Geometry check sheet. Reference: drawing and pictorial views, mm from the part's lowest x, y, z. Round coordinates to 2 decimals unless told otherwise and drop trailing zeros. Write each loop counter-clockwise with the first axis right and the second up, starting at its lowest first coordinate (ties: lowest second). Pieces come first, ordered by that corner, then holes. Notation, with made-up numbers: (83, 64) - (138, 64) arc R21 ccw to (138, 83) - close; hole circle Ø6 at (10, -38). An arc over 180 degrees is marked (long way). Return JSON: item names as keys, results as strings.
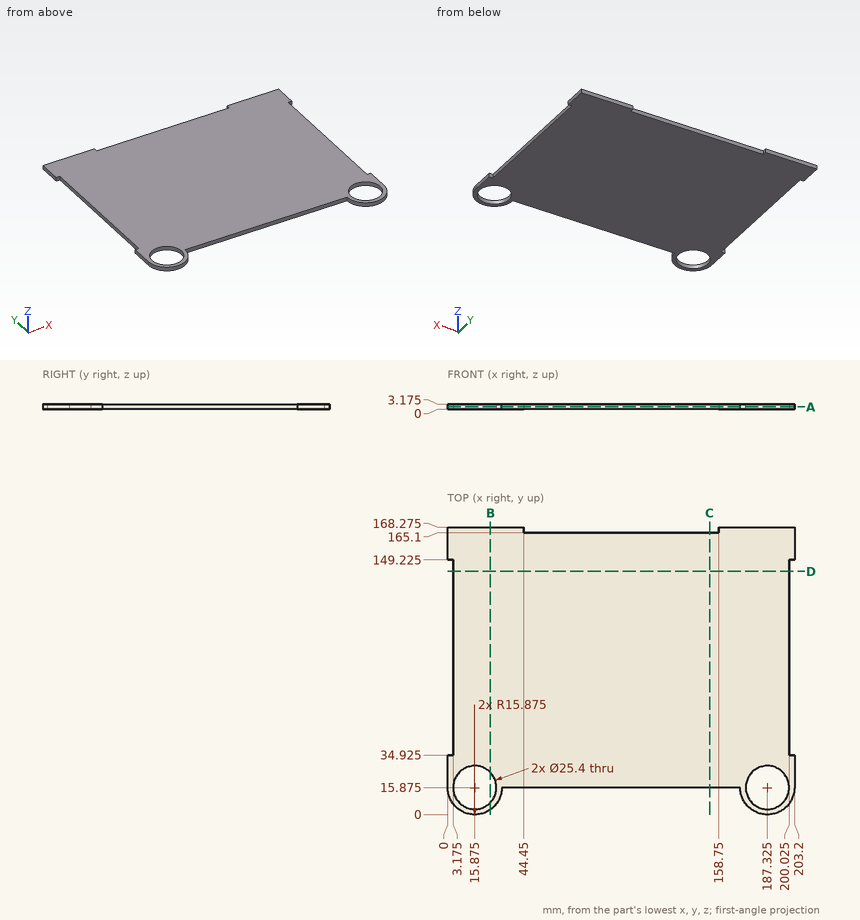
(1) Section check B-B, the plane x = 25. Enter the section's corners in (y, z) (3 decimals).
Response values:
{"outline": "(2.885, 0) - (7.042, 0) - (7.042, 3.175) - (2.885, 3.175) - close; (24.708, 0) - (168.275, 0) - (168.275, 3.175) - (24.708, 3.175) - close"}
(2) Section check A-A, the plane z = 1.45. Enter the section's corners in (x, y) (3 decimals), plus the area to 3 significant figures.
Response values:
{"outline": "(0, 15.875) arc R15.875 ccw to (31.75, 15.875) - (171.45, 15.875) arc R15.875 ccw to (203.2, 15.875) - (203.2, 34.925) - (200.025, 34.925) - (200.025, 149.225) - (203.2, 149.225) - (203.2, 168.275) - (158.75, 168.275) - (158.75, 165.1) - (44.45, 165.1) - (44.45, 168.275) - (0, 168.275) - (0, 149.225) - (3.175, 149.225) - (3.175, 34.925) - (0, 34.925) - close; hole circle Ø25.4 at (15.875, 15.875); hole circle Ø25.4 at (187.325, 15.875)", "area": "29,700 mm^2"}
(3) Section check C-C, the plane x = 153.5. Enter the section's corners in (y, z) (3 decimals), plus the area to 3 significant figures.
Response values:
{"outline": "(15.875, 0) - (165.1, 0) - (165.1, 3.175) - (15.875, 3.175) - close", "area": "474 mm^2"}
(4) Section check D-D, the plane y = 142.5. Enter the section's corners in (x, z) (3 decimals), plus the area to 3 significant figures.
Response values:
{"outline": "(3.175, 0) - (200.025, 0) - (200.025, 3.175) - (3.175, 3.175) - close", "area": "625 mm^2"}
(5) Gauge pin test, flat ends, axial feed: pin 1 (20.5 mm diameter, centred on x = 187.325, y = 15.875, fed in from +Z); pin 2 (1.5 mm diameter, centred on x = 164.5, z = 1.5, fed in from -Y) (3 decimals); pin 3 (1 mm diameter, centred on x = 104.5, z = 2, fed in from +Y); pin 4 (1.6 mm diameter, centred on y = 70, z = 1.5, fed in from -X) (3 decimals). Record the tip position at first contact, or that the pin passes through.
Response values:
{"pin 1": "passes through", "pin 2": "stops at y = 15.875", "pin 3": "stops at y = 165.1", "pin 4": "stops at x = 3.175"}
(6) Material ranges on line 1 along Y through (x, z) = (160, 1.7) (3 decimals); line 2 along X through (y, z) = (136, 2.25) (3 decimals); line 3 along Y through (x, z) = (72, 0.5) (3 decimals), recorded low to high. Write a range as [from, to].
Response values:
{"line 1": "y = [15.875, 168.275]", "line 2": "x = [3.175, 200.025]", "line 3": "y = [15.875, 165.1]"}
